```python
from build123d import *

# Parameters (mm, degrees)
EXTRUSION_DENTS_DEPTH         = 3
R_P_TITION_CIRCULAIRE2_COUNT  = 20
ESQUISSE1_R                   = 8.75
EXTRUSION_DISQUE_DEPTH        = 3
BOSS_EXTRU_1_DEPTH            = 3
ESQUISSE6_R                   = 1.5
BOSS_EXTRU_2_DEPTH            = 3
ESQUISSE3_R                   = 2.35
ENL_V_MAT_EXTRU_1_DEPTH       = 35.263364496
ESQUISSE8_R                   = 0.8
FIXATION_PALONNIER_SG90_DEPTH = 2.5


with BuildPart() as part:
    # Esquisse2 → Extrusion dents (new body)
    with BuildSketch(Plane.XY):
        with BuildLine():
            Line((0, 9.396926208), (0, 8.75))
            ThreePointArc((0, 8.75), (0.761630034, 8.716789529), (1.517478561, 8.617410215))
            Line((1.517478561, 8.617410215), (1.629672464, 9.254533474))
            ThreePointArc((1.629672464, 9.254533474), (1.517874028, 10.109272502), (1.250299377, 10.928712251))
            ThreePointArc((1.250299377, 10.928712251), (0.956235935, 10.958358127), (0.661482168, 10.980092957))
            ThreePointArc((0.661482168, 10.980092957), (0.25763458, 10.219055101), (0, 9.396926208))
        make_face()
    extrude(amount=EXTRUSION_DENTS_DEPTH)


with BuildPart() as r_p_tition_circulaire2_1:
    # R_p_tition circulaire2: pattern copy
    add(part.part.rotate(Axis((0, 0, 0), (0, 0, 1)), 1 * 360 / R_P_TITION_CIRCULAIRE2_COUNT))


with BuildPart() as r_p_tition_circulaire2_2:
    # R_p_tition circulaire2: pattern copy
    add(part.part.rotate(Axis((0, 0, 0), (0, 0, 1)), 2 * 360 / R_P_TITION_CIRCULAIRE2_COUNT))


with BuildPart() as r_p_tition_circulaire2_3:
    # R_p_tition circulaire2: pattern copy
    add(part.part.rotate(Axis((0, 0, 0), (0, 0, 1)), 3 * 360 / R_P_TITION_CIRCULAIRE2_COUNT))


with BuildPart() as r_p_tition_circulaire2_4:
    # R_p_tition circulaire2: pattern copy
    add(part.part.rotate(Axis((0, 0, 0), (0, 0, 1)), 4 * 360 / R_P_TITION_CIRCULAIRE2_COUNT))


with BuildPart() as r_p_tition_circulaire2_5:
    # R_p_tition circulaire2: pattern copy
    add(part.part.rotate(Axis((0, 0, 0), (0, 0, 1)), 5 * 360 / R_P_TITION_CIRCULAIRE2_COUNT))


with BuildPart() as r_p_tition_circulaire2_6:
    # R_p_tition circulaire2: pattern copy
    add(part.part.rotate(Axis((0, 0, 0), (0, 0, 1)), 6 * 360 / R_P_TITION_CIRCULAIRE2_COUNT))


with BuildPart() as r_p_tition_circulaire2_7:
    # R_p_tition circulaire2: pattern copy
    add(part.part.rotate(Axis((0, 0, 0), (0, 0, 1)), 7 * 360 / R_P_TITION_CIRCULAIRE2_COUNT))


with BuildPart() as r_p_tition_circulaire2_8:
    # R_p_tition circulaire2: pattern copy
    add(part.part.rotate(Axis((0, 0, 0), (0, 0, 1)), 8 * 360 / R_P_TITION_CIRCULAIRE2_COUNT))


with BuildPart() as r_p_tition_circulaire2_9:
    # R_p_tition circulaire2: pattern copy
    add(part.part.rotate(Axis((0, 0, 0), (0, 0, 1)), 9 * 360 / R_P_TITION_CIRCULAIRE2_COUNT))


with BuildPart() as r_p_tition_circulaire2_10:
    # R_p_tition circulaire2: pattern copy
    add(part.part.rotate(Axis((0, 0, 0), (0, 0, 1)), 10 * 360 / R_P_TITION_CIRCULAIRE2_COUNT))


with BuildPart() as r_p_tition_circulaire2_11:
    # R_p_tition circulaire2: pattern copy
    add(part.part.rotate(Axis((0, 0, 0), (0, 0, 1)), 11 * 360 / R_P_TITION_CIRCULAIRE2_COUNT))


with BuildPart() as r_p_tition_circulaire2_12:
    # R_p_tition circulaire2: pattern copy
    add(part.part.rotate(Axis((0, 0, 0), (0, 0, 1)), 12 * 360 / R_P_TITION_CIRCULAIRE2_COUNT))


with BuildPart() as r_p_tition_circulaire2_13:
    # R_p_tition circulaire2: pattern copy
    add(part.part.rotate(Axis((0, 0, 0), (0, 0, 1)), 13 * 360 / R_P_TITION_CIRCULAIRE2_COUNT))


with BuildPart() as r_p_tition_circulaire2_14:
    # R_p_tition circulaire2: pattern copy
    add(part.part.rotate(Axis((0, 0, 0), (0, 0, 1)), 14 * 360 / R_P_TITION_CIRCULAIRE2_COUNT))


with BuildPart() as r_p_tition_circulaire2_15:
    # R_p_tition circulaire2: pattern copy
    add(part.part.rotate(Axis((0, 0, 0), (0, 0, 1)), 15 * 360 / R_P_TITION_CIRCULAIRE2_COUNT))


with BuildPart() as r_p_tition_circulaire2_16:
    # R_p_tition circulaire2: pattern copy
    add(part.part.rotate(Axis((0, 0, 0), (0, 0, 1)), 16 * 360 / R_P_TITION_CIRCULAIRE2_COUNT))


with BuildPart() as r_p_tition_circulaire2_17:
    # R_p_tition circulaire2: pattern copy
    add(part.part.rotate(Axis((0, 0, 0), (0, 0, 1)), 17 * 360 / R_P_TITION_CIRCULAIRE2_COUNT))


with BuildPart() as r_p_tition_circulaire2_18:
    # R_p_tition circulaire2: pattern copy
    add(part.part.rotate(Axis((0, 0, 0), (0, 0, 1)), 18 * 360 / R_P_TITION_CIRCULAIRE2_COUNT))


with BuildPart() as r_p_tition_circulaire2_19:
    # R_p_tition circulaire2: pattern copy
    add(part.part.rotate(Axis((0, 0, 0), (0, 0, 1)), 19 * 360 / R_P_TITION_CIRCULAIRE2_COUNT))


with BuildPart() as part_1:
    add(part.part)

    add(r_p_tition_circulaire2_1.part)  # Extrusion disque merges R_p_tition circulaire2_1

    add(r_p_tition_circulaire2_2.part)  # Extrusion disque merges R_p_tition circulaire2_2

    add(r_p_tition_circulaire2_3.part)  # Extrusion disque merges R_p_tition circulaire2_3

    add(r_p_tition_circulaire2_4.part)  # Extrusion disque merges R_p_tition circulaire2_4

    add(r_p_tition_circulaire2_5.part)  # Extrusion disque merges R_p_tition circulaire2_5

    add(r_p_tition_circulaire2_6.part)  # Extrusion disque merges R_p_tition circulaire2_6

    add(r_p_tition_circulaire2_7.part)  # Extrusion disque merges R_p_tition circulaire2_7

    add(r_p_tition_circulaire2_8.part)  # Extrusion disque merges R_p_tition circulaire2_8

    add(r_p_tition_circulaire2_9.part)  # Extrusion disque merges R_p_tition circulaire2_9

    add(r_p_tition_circulaire2_10.part)  # Extrusion disque merges R_p_tition circulaire2_10

    add(r_p_tition_circulaire2_11.part)  # Extrusion disque merges R_p_tition circulaire2_11

    add(r_p_tition_circulaire2_12.part)  # Extrusion disque merges R_p_tition circulaire2_12

    add(r_p_tition_circulaire2_13.part)  # Extrusion disque merges R_p_tition circulaire2_13

    add(r_p_tition_circulaire2_14.part)  # Extrusion disque merges R_p_tition circulaire2_14

    add(r_p_tition_circulaire2_15.part)  # Extrusion disque merges R_p_tition circulaire2_15

    add(r_p_tition_circulaire2_16.part)  # Extrusion disque merges R_p_tition circulaire2_16

    add(r_p_tition_circulaire2_17.part)  # Extrusion disque merges R_p_tition circulaire2_17

    add(r_p_tition_circulaire2_18.part)  # Extrusion disque merges R_p_tition circulaire2_18

    add(r_p_tition_circulaire2_19.part)  # Extrusion disque merges R_p_tition circulaire2_19
    # Esquisse1 → Extrusion disque (add)
    with BuildSketch(Plane.XY):
        Circle(ESQUISSE1_R)
    extrude(amount=EXTRUSION_DISQUE_DEPTH)

    # Esquisse5 → Boss.-Extru.1 (add)
    with BuildSketch(Plane(origin=(0, 0, 0), x_dir=(-1, 0, 0), z_dir=(0, 0, -1))):
        with BuildLine():
            Line((-0.957126431, 10.958280385), (0.957449481, -10.958252164))
            ThreePointArc((0.957449481, -10.958252164), (-10.958266276, -0.957287956), (-0.957126431, 10.958280385))
        make_face()
    extrude(amount=-BOSS_EXTRU_1_DEPTH)

    # Esquisse6 → Boss.-Extru.2 (add)
    with BuildSketch(Plane(origin=(0, 0, 0), x_dir=(-1, 0, 0), z_dir=(0, 0, -1))):
        with BuildLine():
            Line((-7.447050229, -8.095766974), (-17.287454672, -25.507442378))
            ThreePointArc((-17.287454672, -25.507442378), (-16.341045802, -28.913952359), (-12.934535821, -27.967543489))
            Line((-12.934535821, -27.967543489), (-3.094131377, -10.555868085))
            ThreePointArc((-3.094131377, -10.555868085), (-5.412222444, -9.576421473), (-7.447050229, -8.095766974))
        make_face()
        with Locations((-15.110995246, -26.737492934)):
            Circle(ESQUISSE6_R, mode=Mode.SUBTRACT)
    extrude(amount=-BOSS_EXTRU_2_DEPTH)

    # Esquisse3 → Enl_v. mat.-Extru.1 (cut, through all)
    with BuildSketch(Plane.XY.offset(3)):
        Circle(ESQUISSE3_R)
    extrude(amount=-ENL_V_MAT_EXTRU_1_DEPTH, mode=Mode.SUBTRACT)

    # Esquisse8 → Fixation palonnier SG90 (cut)
    with BuildSketch(Plane.XY):
        with Locations((-1.63779007, 5.040599536)):
            Circle(ESQUISSE8_R)
        with Locations((-5.3, 0)):
            Circle(ESQUISSE8_R)
        with Locations((-1.63779007, -5.040599536)):
            Circle(ESQUISSE8_R)
        with Locations((4.28779007, 3.115261837)):
            Circle(ESQUISSE8_R)
        with Locations((4.28779007, -3.115261837)):
            Circle(ESQUISSE8_R)
    extrude(amount=FIXATION_PALONNIER_SG90_DEPTH, mode=Mode.SUBTRACT)


solid = part_1.part
```
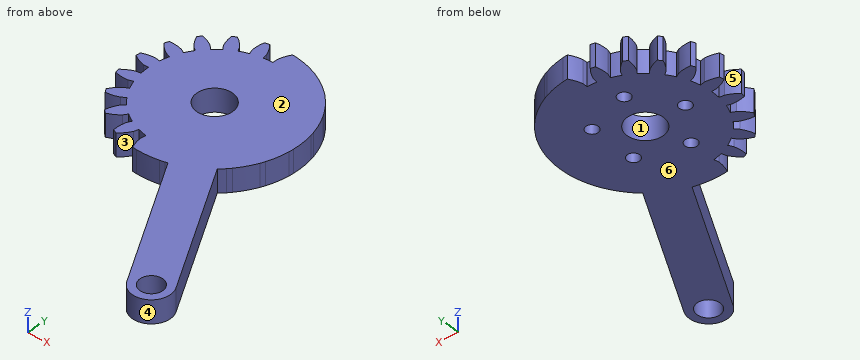
Check sheet for the modelled part. Datum: model origin and axes. Units: mm. Face numbers are marked on the shaded views. A direction names the side the tool comes from. Coordinates: 2 decimals unless noted, no trailing zeros. Loops run counter-clockwise (first coordinate to the right, second up) from the corner with the lowest first, then second, coordinate; pieces in that order, holes last.
1) Sectioned sample at B-B (z = 0.8). Count the separate pieces of the cut face and the enclosed holes in it, and give its area (3 significant figures).
2) Sectioned sample at A-A (x = 15.5). Record the boundary of the cut face in (y, z).
3) Material ranges on probe 1 along Y at (x, z) = (-5.3, 0.9); probe 2 along Y at (x, z) = (-2, 0.25); probe 3 along X at (y, z) = (9.5, 1.3), recorded low to high.
4) Access from +Z, -Z, +X, -X, +Y, -Y to the whole of each face (thin tool, end or side, straight path). Record for the marked faces 5 and 6.
5) Gauge pin test, flat ends, axial feed: pin 1 (0.8 mm diameter, centred on x = 4, y = -3.5, fed in from -Z); pin 2 (8 mm diameter, centred on x = 14.5, y = -6, fed in from +Z); pin 3 (0.8 mm diameter, centred on x = -1.5, y = 5, fed in from -Z); pin 4 (0.5 mm diameter, centred on y = 9, z = 1, fed in from -X). Record the tip position at first contact, or that the pin passes through.
6) Release check for a two-part mould opening along Y. For the marked faces 1, 2, 3 and 4 record: released by +Y, released by -Y, zero draft, split by the parting line, or undercut.
7) Sectioned sample at C-C (y = -12). Record the boundary of the cut face in (x, z), and give its area (3 significant figures).
Check sheet entries:
1. separate pieces: 1
1. enclosed holes: 7
1. area: 415 mm2
2. outline: (-29.21, 0) - (-28.19, 0) - (-28.19, 3) - (-29.21, 3) - close; (-25.29, 0) - (-22.34, 0) - (-22.34, 3) - (-25.29, 3) - close
3. probe 1: y = -7.29 to -0.8, 0.8 to 6.96, 7.29 to 9.51
3. probe 2: y = -8.52 to -5.75, -4.33 to -1.23, 1.23 to 4.33, 5.75 to 10.55
3. probe 3: x = -5.55 to -5.29, -2.93 to -1.39, 0.02 to 5.55
4. face 5: +Z, -Z, -X
4. face 6: -Z, +X, -X, +Y, -Y
5. pin 1: stops at z = 0
5. pin 2: passes through
5. pin 3: stops at z = 2.5
5. pin 4: stops at x = -5.92
6. face 1: undercut
6. face 2: zero draft
6. face 3: released by -Y
6. face 4: split by the parting line
7. outline: (3.91, 0) - (9.65, 0) - (9.65, 3) - (3.91, 3) - close
7. area: 17.2 mm2
